For this review, use the dimensioned drawing (mm, ordinates from the lowest corner) and the shaded views. A direction names the side the tool comes from. Round coordinates to 2 decimals unless told otherwise and drop trailing zeros. Write each loop counter-clockwise with the first axis right and the second up, starting at its lowest first coordinate (ties: lowest second). Pieces come first, ordered by that corner, then holes. Notation, with made-up numbers: M 2,4 L 48,4 A25 cw 48,23 Z; hole C 37,29 d3. An arc over 180 degrees is marked long. Answer in a Markdown table with one row per item.
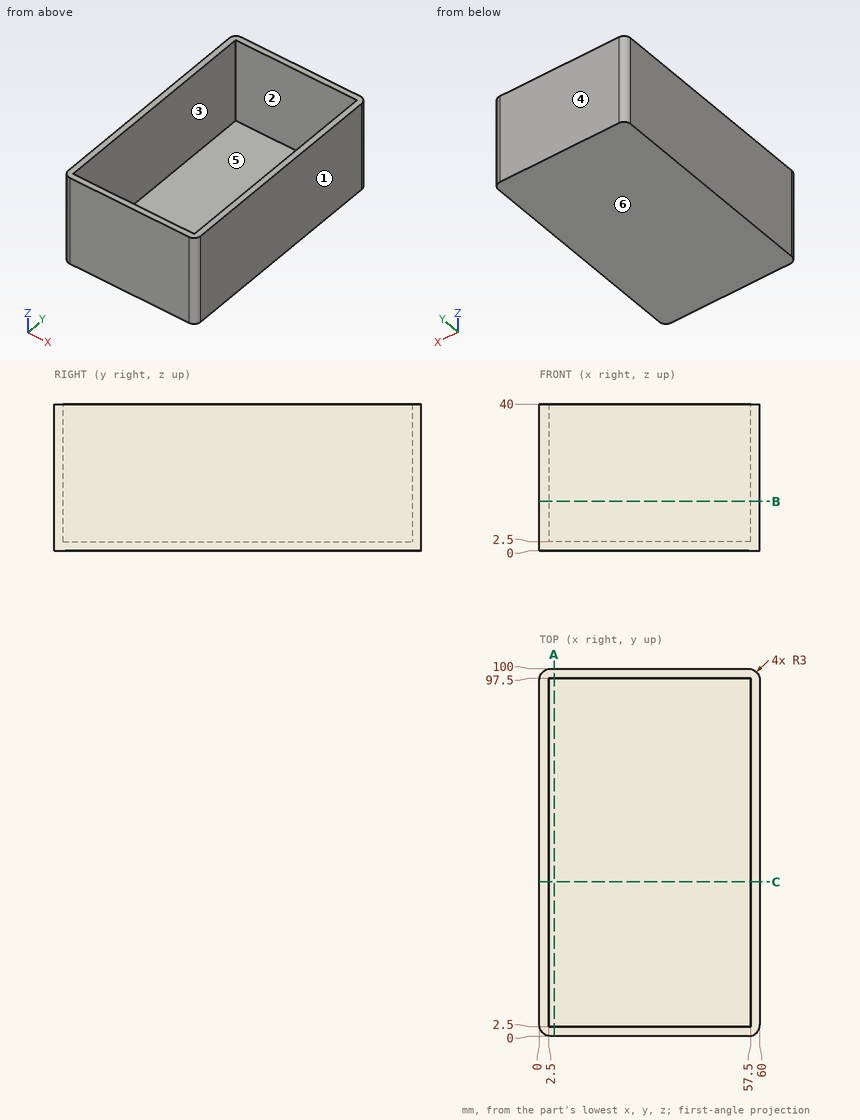
Q1. Take a section at C-C (y = 42). State the section outline as (x, z) points.
Found:
| item | result |
|---|---|
| outline | M 0,0 L 60,0 L 60,40 L 57.5,40 L 57.5,2.5 L 2.5,2.5 L 2.5,40 L 0,40 Z |
Q2. Mouldability with a two-part tool opening along X and no side actions: class the marked faces 1, 2, 3 and 4 as +X half, -X half, draft (parallel to the pull), parting line (faces both ways), or undercut.
Found:
| item | result |
|---|---|
| face 1 | +X half |
| face 2 | undercut |
| face 3 | undercut |
| face 4 | draft |
Q3. Machinability: for the marked faces 5 and 6, which of the approach directions +Z, -Z, +X, -X, +Y, -Y give a long, thin tool a straight path to every point of the face, cutting with its end or side? Answer none if there is none.
Found:
| item | result |
|---|---|
| face 5 | +Z |
| face 6 | -Z, +X, -X, +Y, -Y |
Q4. Take a section at A-A (x = 4). State the section outline as (y, z) points, then the cut area to 4 significant figures.
Found:
| item | result |
|---|---|
| outline | M 0,0 L 100,0 L 100,40 L 97.5,40 L 97.5,2.5 L 2.5,2.5 L 2.5,40 L 0,40 Z |
| area | 437.5 mm² |
Q5. For probe 1 along X at (y, z) = (73, 3); probe 2 along Y at (x, z) = (30.5, 25.5); probe 3 along Z at (x, y) = (55.5, 66.5), list the stretches that pass through material, from the lowest coordinate up.
Found:
| item | result |
|---|---|
| probe 1 | 0 to 2.5, 57.5 to 60 |
| probe 2 | 0 to 2.5, 97.5 to 100 |
| probe 3 | 0 to 2.5 |
Q6. Take a section at B-B (z = 13.5). State the section outline as (x, y) points.
Found:
| item | result |
|---|---|
| outline | M 0,3 A3 ccw 3,0 L 57,0 A3 ccw 60,3 L 60,97 A3 ccw 57,100 L 3,100 A3 ccw 0,97 Z; hole M 2.5,2.5 L 57.5,2.5 L 57.5,97.5 L 2.5,97.5 Z |
Q7. Insertion check: P1, Ø16.5, axis at x = 36.5, y = 37.5, coming from the +Z side. The pin has a flat end and moves straight along its axis. Give the tip position at first contact, or say it passes through.
Found:
| item | result |
|---|---|
| P1 | z = 2.5 |
